Check sheet for the modelled part. Datum: model origin and axes. Units: mm. Face numbers are marked on the shaded views. Coordinates: 2 decimals unless noted, no trailing zeros. Write each loop counter-clockwise with the first axis right and the second up, starting at its lowest first coordinate (ties: lowest second). Pieces come first, ordered by that corner, then holes. Notation, with made-up numbers: (-11, 45.5) - (5, 45.5) arc R26 ccw to (5, 64.5) - close; hole circle Ø11 at (60.5, -20.75). An arc over 180 degrees is marked (long way). Answer as CSV lines item,"result". Start each with the question number.
from build123d import *

# Parameters (mm, degrees)
BOSS_EXTRUDE1_DEPTH = 5
SKETCH4_R           = 1.5
CUT_EXTRUDE1_DEPTH  = 5


with BuildPart() as part:
    # Sketch2 → Boss-Extrude1 (new body)
    with BuildSketch(Plane.XY):
        with BuildLine():
            Line((-75, 15), (75, 15))
            ThreePointArc((75, 15), (90, 0), (75, -15))
            Line((75, -15), (-75, -15))
            ThreePointArc((-75, -15), (-90, 0), (-75, 15))
        make_face()
    extrude(amount=BOSS_EXTRUDE1_DEPTH)

    # Sketch4 → Cut-Extrude1 (cut)
    with BuildSketch(Plane(origin=(0, 0, 0), x_dir=(-1, 0, 0), z_dir=(0, 0, -1))):
        with Locations((-75, 0)):
            Circle(SKETCH4_R)
        with BuildLine():
            Line((44.583333333, 4.982608643), (74.375, 7.473912964))
            ThreePointArc((74.375, 7.473912964), (82.5, 0), (74.375, -7.473912964))
            Line((74.375, -7.473912964), (44.583333333, -4.982608643))
            ThreePointArc((44.583333333, -4.982608643), (40, 0), (44.583333333, 4.982608643))
        make_face()
    extrude(amount=-CUT_EXTRUDE1_DEPTH, mode=Mode.SUBTRACT)


solid = part.part
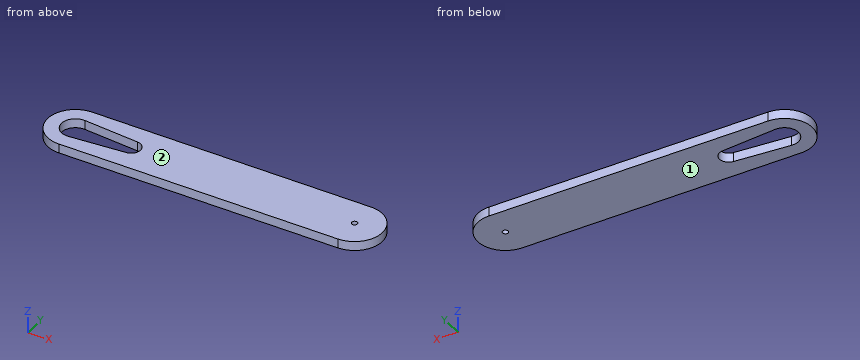
(1) Cross-section at C-C on x = -59. Record the boundary of the cut face in (y, z).
(2) Cross-section at A-A on y = 0. Record the boundary of the cut face in (x, z), plus the area to 4 significant figures.
(3) Material ranges on probe 1 along Y at (x, z) = (75, 1.8); probe 2 along Y at (x, z) = (-75, 2.6); probe 3 along X at (y, z) = (4, 4.7), recorded low to high. Write a range as from..to.
(4) Cross-section at D-D on y = 12.5. Record the boundary of the cut face in (x, z), plus the area to 3 significant figures.
(5) Go/stop test with flat-tipped pins: P1, Ø8, axis at x = 63, y = -10, coming from the -Z side; P2, Ø9, axis at x = -75, y = 0, coming from the +Z side. Record where each tip stops, or that it passes through.
(6) Release check for a two-part mould opening along Z. For the marked faces 1 and 2 record: pulls with the +Z half, pulls with the -Z half, needs draft (parallel to the pull), parting line crosses it, or undercut.
(7) Cross-section at B-B on z = 2.8. Record the boundary of the cut face in (x, y) (3 decimals), plus the area to 3 significant figures.
Checked values:
1,outline,"(-15, 0) - (-6.19, 0) - (-6.19, 5) - (-15, 5) - close; (6.19, 0) - (15, 0) - (15, 5) - (6.19, 5) - close"
2,outline,"(-90, 0) - (-82.5, 0) - (-82.5, 5) - (-90, 5) - close; (-40, 0) - (73.5, 0) - (73.5, 5) - (-40, 5) - close; (76.5, 0) - (90, 0) - (90, 5) - (76.5, 5) - close"
2,area,"672.5 mm^2"
3,probe 1,"-15..-1.5, 1.5..15"
3,probe 2,"-15..-7.5, 7.5..15"
3,probe 3,"-89.46..-81.34, -42..89.46"
4,outline,"(-83.29, 0) - (83.29, 0) - (83.29, 5) - (-83.29, 5) - close"
4,area,"833 mm^2"
5,P1,"z = 0"
5,P2,"through"
6,face 1,"pulls with the -Z half"
6,face 2,"pulls with the +Z half"
7,outline,"(-75, -15) - (75, -15) arc R15 ccw to (75, 15) - (-75, 15) arc R15 ccw to start; hole (-74.375, -7.474) - (-44.583, -4.983) arc R5 ccw to (-44.583, 4.983) - (-74.375, 7.474) arc R7.5 ccw (long way) to start; hole circle Ø3 at (75, 0)"
7,area,"4,700 mm^2"
